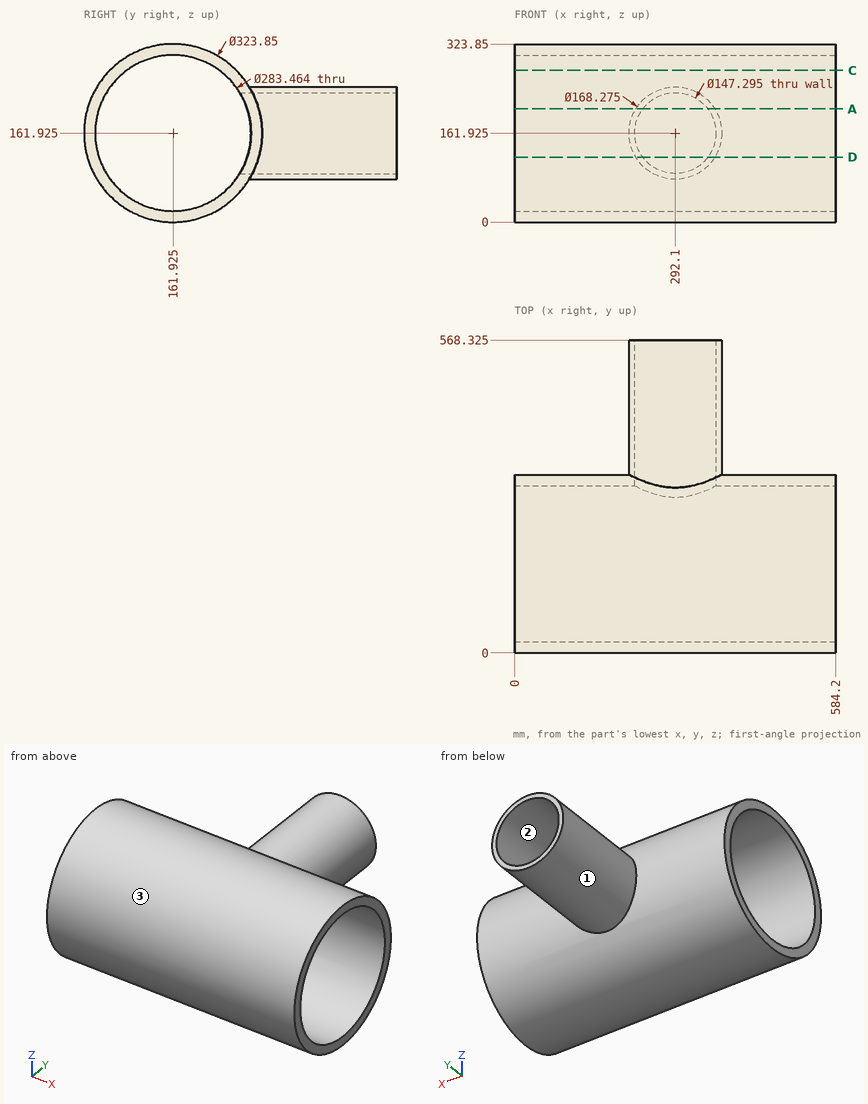
Check sheet for the drawn part. Datum: minimum x, y, z corner. Units: mm. Round coordinates to 2 decimals unless told otherwise and drop trailing zeros. Order: outer loops, then holes, each group sorted by start corner. A loop starts at its lowest first (then second) coordinate and runs counter-clockwise, first axis right, second up.
1) Go/stop test with flat-tipped pins: pin 1 Ø12 at (y, z) = (330, 201) entering from -X; pin 2 Ø2 at (x, z) = (170, 38) entering from +Y (1 decimal); pin 3 Ø1.5 at (x, z) = (300, 169) entering from -Y. Record where each tip stops, or that it passes through.
2) Section check A-A (z = 206). Record the boundary of the cut face in (x, y) (1 decimal).
3) Mould release check, pull along X, two halves, no side actions. Record for the marked faces 1, 2 and 3: +X half, -X half, draft (parallel to the pull), parting line (faces both ways), or undercut.
4) Section check D-D (z = 118). Record the boundary of the cut face in (x, y) (1 decimal), and give its area (3 significant figures).
5) Section check C-C (z = 276). Record the boundary of the cut face in (x, y) (1 decimal), and give its area (3 significant figures).
6) Scan lines: line 1 (Z direction, x = 292, y = 371); line 2 (Y direction, x = 492.5, z = 49.5); line 3 (Y direction, x = 364, z = 96). Record each from-to range of solid material in increasing order.
Result:
1. pin 1: stops at x = 214.74
1. pin 2: stops at y = 267.3
1. pin 3: stops at y = 0.12
2. outline: (0, 6.1) - (584.2, 6.1) - (584.2, 27.2) - (0, 27.2) - close; (0, 296.6) - (233.1, 296.6) - (233.1, 568.3) - (220.4, 568.3) - (220.4, 317.7) - (0, 317.7) - close; (351.1, 296.6) - (584.2, 296.6) - (584.2, 317.7) - (363.8, 317.7) - (363.8, 568.3) - (351.1, 568.3) - close
3. face 1: parting line
3. face 2: undercut
3. face 3: draft
4. outline: (0, 6.1) - (584.2, 6.1) - (584.2, 27.2) - (0, 27.2) - close; (0, 296.7) - (233, 296.7) - (233, 568.3) - (220.3, 568.3) - (220.3, 317.8) - (0, 317.8) - close; (351.2, 296.7) - (584.2, 296.7) - (584.2, 317.8) - (363.9, 317.8) - (363.9, 568.3) - (351.2, 568.3) - close
4. area: 28,500 mm2
5. outline: (0, 47) - (584.2, 47) - (584.2, 77.8) - (0, 77.8) - close; (0, 246) - (584.2, 246) - (584.2, 276.8) - (0, 276.8) - close
5. area: 36,000 mm2
6. line 1: z = 77.79 to 88.28, 235.57 to 246.06
6. line 2: y = 45.39 to 75.62, 248.23 to 278.46
6. line 3: y = 14.03 to 36.46, 287.39 to 309.82
